Read the model definition and answer for the solid it produces. Units are mm, in the model's axes. A direction names the side the tool comes from. Coordinates: 2 decimals unless noted, no trailing zeros. Order: outer loops, then holes, each group sorted by start corner. A loop starts at its lowest first (then second) coordinate and runs counter-clockwise, first axis right, second up.
```python
from build123d import *

# Parameters (mm, degrees)
SKETCH1_W          = 174
SKETCH1_H          = 154.7
SKETCH1_R          = 1.575
BASE_FLANGE1_DEPTH = 1.5
FILLET1_R          = 2
CUT_EXTRUDE1_DEPTH = 117.422817781
SKETCH7_R          = 6
TAB1_DEPTH         = 1.5
SKETCH10_R         = 3.15
CUT_EXTRUDE2_DEPTH = 120.117893282
FILLET2_R          = 3


# Sheet-metal steps are written as plain solids
with BuildPart() as part:
    # Sketch1 → Base-Flange1 (new body)
    with BuildSketch(Plane(origin=(0, 0, 0), x_dir=(1, 0, 0), z_dir=(0, 1, 0))):
        Rectangle(SKETCH1_W, SKETCH1_H)
        with Locations(Location((-79, 72.85, 0), (0, 0, 270))):
            Circle(SKETCH1_R, mode=Mode.SUBTRACT)
        with Locations(Location((79, 72.85, 0), (0, 0, 270))):
            Circle(SKETCH1_R, mode=Mode.SUBTRACT)
        with Locations(Location((79, -72.85, 0), (0, 0, 270))):
            Circle(SKETCH1_R, mode=Mode.SUBTRACT)
        with Locations(Location((-79, -72.85, 0), (0, 0, 270))):
            Circle(SKETCH1_R, mode=Mode.SUBTRACT)
    extrude(amount=-BASE_FLANGE1_DEPTH)

    # Fillet1
    fillet1_edges = [part.edges().sort_by_distance(p)[0] for p in [
        (-87, -0.75, -77.35),
        (87, -0.75, -77.35),
        (87, -0.75, 77.35),
        (-87, -0.75, 77.35),
    ]]
    fillet(fillet1_edges, radius=FILLET1_R)

    # Sketch6 → Cut-Extrude1 (cut, through all)
    with BuildSketch(Plane(origin=(0, 0, 0), x_dir=(1, 0, 0), z_dir=(0, 1, 0))):
        with BuildLine():
            Line((26.529437252, -66.057106781), (61.884776311, -30.701767722))
            ThreePointArc((61.884776311, -30.701767722), (61.884776311, -29.287554159), (60.470562748, -29.287554159))
            Line((60.470562748, -29.287554159), (25.115223689, -64.642893219))
            ThreePointArc((25.115223689, -64.642893219), (25.115223689, -66.057106781), (26.529437252, -66.057106781))
        make_face()
        with BuildLine():
            Line((26.529437252, -56.522640687), (61.884776311, -21.167301628))
            ThreePointArc((61.884776311, -21.167301628), (61.884776311, -19.753088065), (60.470562748, -19.753088065))
            Line((60.470562748, -19.753088065), (25.115223689, -55.108427125))
            ThreePointArc((25.115223689, -55.108427125), (25.115223689, -56.522640687), (26.529437252, -56.522640687))
        make_face()
        with BuildLine():
            Line((26.529437252, -46.988174593), (61.884776311, -11.632835534))
            ThreePointArc((61.884776311, -11.632835534), (61.884776311, -10.218621971), (60.470562748, -10.218621971))
            Line((60.470562748, -10.218621971), (25.115223689, -45.573961031))
            ThreePointArc((25.115223689, -45.573961031), (25.115223689, -46.988174593), (26.529437252, -46.988174593))
        make_face()
        with BuildLine():
            Line((26.529437252, -37.453708499), (61.884776311, -2.09836944))
            ThreePointArc((61.884776311, -2.09836944), (61.884776311, -0.684155877), (60.470562748, -0.684155877))
            Line((60.470562748, -0.684155877), (25.115223689, -36.039494937))
            ThreePointArc((25.115223689, -36.039494937), (25.115223689, -37.453708499), (26.529437252, -37.453708499))
        make_face()
        with BuildLine():
            Line((26.529437252, -27.919242405), (61.884776311, 7.436096654))
            ThreePointArc((61.884776311, 7.436096654), (61.884776311, 8.850310217), (60.470562748, 8.850310217))
            Line((60.470562748, 8.850310217), (25.115223689, -26.505028843))
            ThreePointArc((25.115223689, -26.505028843), (25.115223689, -27.919242405), (26.529437252, -27.919242405))
        make_face()
        with BuildLine():
            Line((26.529437252, -18.384776311), (61.884776311, 16.970562748))
            ThreePointArc((61.884776311, 16.970562748), (61.884776311, 18.384776311), (60.470562748, 18.384776311))
            Line((60.470562748, 18.384776311), (25.115223689, -16.970562748))
            ThreePointArc((25.115223689, -16.970562748), (25.115223689, -18.384776311), (26.529437252, -18.384776311))
        make_face()
        with BuildLine():
            Line((26.529437252, -8.850310217), (61.884776311, 26.505028843))
            ThreePointArc((61.884776311, 26.505028843), (61.884776311, 27.919242405), (60.470562748, 27.919242405))
            Line((60.470562748, 27.919242405), (25.115223689, -7.436096654))
            ThreePointArc((25.115223689, -7.436096654), (25.115223689, -8.850310217), (26.529437252, -8.850310217))
        make_face()
        with BuildLine():
            Line((26.529437252, 0.684155877), (61.884776311, 36.039494937))
            ThreePointArc((61.884776311, 36.039494937), (61.884776311, 37.453708499), (60.470562748, 37.453708499))
            Line((60.470562748, 37.453708499), (25.115223689, 2.09836944))
            ThreePointArc((25.115223689, 2.09836944), (25.115223689, 0.684155877), (26.529437252, 0.684155877))
        make_face()
        with BuildLine():
            Line((26.529437252, 10.218621971), (61.884776311, 45.573961031))
            ThreePointArc((61.884776311, 45.573961031), (61.884776311, 46.988174593), (60.470562748, 46.988174593))
            Line((60.470562748, 46.988174593), (25.115223689, 11.632835534))
            ThreePointArc((25.115223689, 11.632835534), (25.115223689, 10.218621971), (26.529437252, 10.218621971))
        make_face()
        with BuildLine():
            Line((26.529437252, 19.753088065), (61.884776311, 55.108427125))
            ThreePointArc((61.884776311, 55.108427125), (61.884776311, 56.522640687), (60.470562748, 56.522640687))
            Line((60.470562748, 56.522640687), (25.115223689, 21.167301628))
            ThreePointArc((25.115223689, 21.167301628), (25.115223689, 19.753088065), (26.529437252, 19.753088065))
        make_face()
        with BuildLine():
            Line((26.529437252, 29.287554159), (61.884776311, 64.642893219))
            ThreePointArc((61.884776311, 64.642893219), (61.884776311, 66.057106781), (60.470562748, 66.057106781))
            Line((60.470562748, 66.057106781), (25.115223689, 30.701767722))
            ThreePointArc((25.115223689, 30.701767722), (25.115223689, 29.287554159), (26.529437252, 29.287554159))
        make_face()
        with BuildLine():
            Line((-25.115223689, 30.701767722), (-60.470562748, 66.057106781))
            ThreePointArc((-60.470562748, 66.057106781), (-61.884776311, 66.057106781), (-61.884776311, 64.642893219))
            Line((-61.884776311, 64.642893219), (-26.529437252, 29.287554159))
            ThreePointArc((-26.529437252, 29.287554159), (-25.115223689, 29.287554159), (-25.115223689, 30.701767722))
        make_face()
        with BuildLine():
            Line((-25.115223689, 21.167301628), (-60.470562748, 56.522640687))
            ThreePointArc((-60.470562748, 56.522640687), (-61.884776311, 56.522640687), (-61.884776311, 55.108427125))
            Line((-61.884776311, 55.108427125), (-26.529437252, 19.753088065))
            ThreePointArc((-26.529437252, 19.753088065), (-25.115223689, 19.753088065), (-25.115223689, 21.167301628))
        make_face()
        with BuildLine():
            Line((-25.115223689, 11.632835534), (-60.470562748, 46.988174593))
            ThreePointArc((-60.470562748, 46.988174593), (-61.884776311, 46.988174593), (-61.884776311, 45.573961031))
            Line((-61.884776311, 45.573961031), (-26.529437252, 10.218621971))
            ThreePointArc((-26.529437252, 10.218621971), (-25.115223689, 10.218621971), (-25.115223689, 11.632835534))
        make_face()
        with BuildLine():
            Line((-25.115223689, 2.09836944), (-60.470562748, 37.453708499))
            ThreePointArc((-60.470562748, 37.453708499), (-61.884776311, 37.453708499), (-61.884776311, 36.039494937))
            Line((-61.884776311, 36.039494937), (-26.529437252, 0.684155877))
            ThreePointArc((-26.529437252, 0.684155877), (-25.115223689, 0.684155877), (-25.115223689, 2.09836944))
        make_face()
        with BuildLine():
            Line((-25.115223689, -7.436096654), (-60.470562748, 27.919242405))
            ThreePointArc((-60.470562748, 27.919242405), (-61.884776311, 27.919242405), (-61.884776311, 26.505028843))
            Line((-61.884776311, 26.505028843), (-26.529437252, -8.850310217))
            ThreePointArc((-26.529437252, -8.850310217), (-25.115223689, -8.850310217), (-25.115223689, -7.436096654))
        make_face()
        with BuildLine():
            Line((-25.115223689, -16.970562748), (-60.470562748, 18.384776311))
            ThreePointArc((-60.470562748, 18.384776311), (-61.884776311, 18.384776311), (-61.884776311, 16.970562748))
            Line((-61.884776311, 16.970562748), (-26.529437252, -18.384776311))
            ThreePointArc((-26.529437252, -18.384776311), (-25.115223689, -18.384776311), (-25.115223689, -16.970562748))
        make_face()
        with BuildLine():
            Line((-25.115223689, -26.505028843), (-60.470562748, 8.850310217))
            ThreePointArc((-60.470562748, 8.850310217), (-61.884776311, 8.850310217), (-61.884776311, 7.436096654))
            Line((-61.884776311, 7.436096654), (-26.529437252, -27.919242405))
            ThreePointArc((-26.529437252, -27.919242405), (-25.115223689, -27.919242405), (-25.115223689, -26.505028843))
        make_face()
        with BuildLine():
            Line((-25.115223689, -36.039494937), (-60.470562748, -0.684155877))
            ThreePointArc((-60.470562748, -0.684155877), (-61.884776311, -0.684155877), (-61.884776311, -2.09836944))
            Line((-61.884776311, -2.09836944), (-26.529437252, -37.453708499))
            ThreePointArc((-26.529437252, -37.453708499), (-25.115223689, -37.453708499), (-25.115223689, -36.039494937))
        make_face()
        with BuildLine():
            Line((-25.115223689, -45.573961031), (-60.470562748, -10.218621971))
            ThreePointArc((-60.470562748, -10.218621971), (-61.884776311, -10.218621971), (-61.884776311, -11.632835534))
            Line((-61.884776311, -11.632835534), (-26.529437252, -46.988174593))
            ThreePointArc((-26.529437252, -46.988174593), (-25.115223689, -46.988174593), (-25.115223689, -45.573961031))
        make_face()
        with BuildLine():
            Line((-25.115223689, -55.108427125), (-60.470562748, -19.753088065))
            ThreePointArc((-60.470562748, -19.753088065), (-61.884776311, -19.753088065), (-61.884776311, -21.167301628))
            Line((-61.884776311, -21.167301628), (-26.529437252, -56.522640687))
            ThreePointArc((-26.529437252, -56.522640687), (-25.115223689, -56.522640687), (-25.115223689, -55.108427125))
        make_face()
        with BuildLine():
            Line((-25.115223689, -64.642893219), (-60.470562748, -29.287554159))
            ThreePointArc((-60.470562748, -29.287554159), (-61.884776311, -29.287554159), (-61.884776311, -30.701767722))
            Line((-61.884776311, -30.701767722), (-26.529437252, -66.057106781))
            ThreePointArc((-26.529437252, -66.057106781), (-25.115223689, -66.057106781), (-25.115223689, -64.642893219))
        make_face()
    extrude(amount=-CUT_EXTRUDE1_DEPTH, mode=Mode.SUBTRACT)

    # Sketch7 → Tab1 (add)
    with BuildSketch(Plane(origin=(0, 0, 0), x_dir=(1, 0, 0), z_dir=(0, 1, 0))):
        with Locations((-50.194998341, 75.35)):
            Circle(SKETCH7_R)
    extrude(amount=-TAB1_DEPTH)

    # Sketch10 → Cut-Extrude2 (cut, through all)
    with BuildSketch(Plane(origin=(0, 0, 0), x_dir=(1, 0, 0), z_dir=(0, 1, 0))):
        with Locations(Location((-50.194998341, 75.35, 0), (0, 0, 270))):
            Circle(SKETCH10_R)
    extrude(amount=-CUT_EXTRUDE2_DEPTH, mode=Mode.SUBTRACT)

    # Fillet2
    fillet2_edges = [part.edges().sort_by_distance(p)[0] for p in [
        (-55.85185259, -0.75, -77.35),
        (-44.538144091, -0.75, -77.35),
    ]]
    fillet(fillet2_edges, radius=FILLET2_R)


solid = part.part
```
1) Which of the six approach directions +Z, -Z, +X, -X, +Y, -Y give full straight-line access (tool end or side, diameter ignored) to faces 3 (the flat face through (-44.455, -0.74, -37.678)), 4 (the flat face through (-1, 0, -3))?
A:
face 3: +Y, -Y
face 4: +Z, -Z, +X, -X, +Y
2) A flat-ended cylindrical pin translates along its axis: pin 1 Ø3 at (x, z) = (79, -72.85) entering from -Y. Find the tip coordinate at first contact, or state that the pin passes through.
A:
pin 1: passes through
3) Straight lines are drawn through the part: line 1 (Z direction, x = 79, y = -1.2) (3 decimals); line 2 (X direction, y = -0.45, z = 72.85) (3 decimals); line 3 (X direction, y = -0.85, z = -72.85) (3 decimals). For each, find the intervals that lie inside material, in ascending order.
A:
line 1: z = -77.35 to -74.425, -71.275 to 71.275, 74.425 to 77.35
line 2: x = -87 to -80.575, -77.425 to 77.425, 80.575 to 87
line 3: x = -87 to -80.575, -77.425 to -52.111, -48.279 to 77.425, 80.575 to 87
4) A cutting plane is placed at B-B, the plane x = 31. State how many separate pieces and enclosed holes the cut face has, and give its area (3 significant figures).
A:
separate pieces: 12
enclosed holes: 0
area: 185 mm2
5) Determine the mould class of faces 1 (the flat face through (-44.455, -0.74, 19.529)), 2 (the flat face through (-1, -1.5, -3)) for opening direction Z: pulls with the +Z half, pulls with the -Z half, needs draft (parallel to the pull), parting line crosses it, or undercut.
A:
face 1: undercut
face 2: needs draft
6) A cutting plane is placed at A-A, the plane x = -9.5. Determine the outline of the cut face in (y, z), and give its area (3 significant figures).
A:
outline: (-1.5, -77.35) - (0, -77.35) - (0, 77.35) - (-1.5, 77.35) - close
area: 232 mm2
